The model under review builds one solid part; all positions refer to its coordinate system, in mm. A direction names the side the tool comes from. Round coordinates to 2 decimals unless told otherwise and drop trailing zeros. Order: outer loops, then holes, each group sorted by start corner. A loop starts at its lowest first (then second) coordinate and runs counter-clockwise, first axis right, second up. Notation, with made-up numbers: M 17,26.5 L 62,26.5 A20 cw 62,55.5 Z; hole C -32.75,77 d7. An arc over 180 degrees is marked long. Use a Markdown table: item, result. Add a question column.
1. Insertion check: P1, Ø1, axis at x = -1, z = 0.5, coming from the +Y side; P2, Ø1, axis at x = 33.5, z = -0.5, coming from the +Y side. Each pin has a flat end and moves straight along its axis. Give the tip position at first contact, or say it passes through.
2. Consider section B-B on x = 10.5. State the section outline as (y, z) points.
3. For faces 4 (the flat face through (25, -45, 0)), 5 (the flat face through (45, -50, 0)), 6 (the flat face through (0, 42, 0)), list the 3-axis set-ups (+Z, -Z, +X, -X, +Y, -Y) from which the entire face can be reached by the end or side of a thin tool; tool diameter is ignored.
4. Consider section A-A on z = -0.7. State the section outline as (x, y) points, then the cut area to 3 significant figures.
5. To check wall thickness, follow probe 1 along X at (y, z) = (30.5, -1); probe 2 along Y at (x, z) = (9, -0.9); probe 3 along Y at (x, z) = (2, -0.3). State the ranges of each line that lie inside material, in increasing order.
6. Consider section C-C on y = 19. State the section outline as (x, z) points, then the cut area to 4 significant figures.
7. The part is to be moulded in two halves that separate along Y. For faces 1 (the flat face through (4, 45, 0)), 2 (the flat face through (5, -1, 0)), 3 (the flat face through (3.146, 43.479, -0.022)), say which applies: +Y half, -Y half, draft (parallel to the pull), parting line (faces both ways), or undercut.
Autodesk Inventor part; units mm, degrees
ref_plane "YZ Plane" through (0, 0, 0) normal (1, 0, 0) x (0, 1, 0)
ref_plane "XZ Plane" through (0, 0, 0) normal (0, 1, 0) x (-1, 0, 0)
ref_plane "XY Plane" through (0, 0, 0) normal (0, 0, 1) x (1, 0, 0)
sketch "Sketch1" plane through (0, 0, 0) normal (0, 0, 1) x (1, 0, 0)
  line L0 (5, -45) -> (5, 45)
  line L1 (-5, 45) -> (-5, -55)
  line L2 (-5, -55) -> (45, -55)
  line L3 (45, -55) -> (45, -45)
  line L4 (45, -45) -> (5, -45)
  line L5 (0, 45) -> (0, 42) construction
  line L6 (0, 42) -> (4, 42)
  line L7 (4, 42) -> (0, 42)
  line L8 (4, 42) -> (11.2559, 42) construction
  line L9 (4, 42) -> (2.2679, 45)
  line L10 (4, 42) -> (7.4641, 42) construction
  line L11 (0, 42) -> (-4, 42)
  line L12 (-4, 42) -> (-2.2679, 45)
  line L13 (-5, 45) -> (-2.2679, 45)
  line L14 (2.2679, 45) -> (5, 45)
  line L15 (2.2679, 45) -> (-2.2679, 45) construction
  point P0 (0, 0)
  dimension "d0" = 10
  dimension "d1" = 45
  dimension "d2" = 100
  dimension "d3" = 45
  dimension "d4" = 5
  dimension "d5" = 50
  dimension "d8" = 3
  dimension "d9" = 4
  dimension "d12" = 120
  dimension "d13" = 4
  dimension "d14" = 60
  dimension "d15" = 45
  dimension "d16" = 87
  dimension "d17" = 33.7441
extrude "Extrusion1" add sketch "Sketch1" along normal mid plane 3.175
properties part number "Liu_Inital_L"
Answer block:
| question | item | result |
|---|---|---|
| 1 | P1 | y = 42 |
| 1 | P2 | y = -45 |
| 2 | outline | M -55,-1.59 L -45,-1.59 L -45,1.59 L -55,1.59 Z |
| 3 | face 4 | +Z, -Z, +X, +Y |
| 3 | face 5 | +Z, -Z, +X, +Y, -Y |
| 3 | face 6 | +Z, -Z |
| 4 | outline | M -5,-55 L 45,-55 L 45,-45 L 5,-45 L 5,45 L 2.27,45 L 4,42 L -4,42 L -2.27,45 L -5,45 Z |
| 4 | area | 1,380 mm^2 |
| 5 | probe 1 | -5 to 5 |
| 5 | probe 2 | -55 to -45 |
| 5 | probe 3 | -55 to 42 |
| 6 | outline | M -5,-1.59 L 5,-1.59 L 5,1.59 L -5,1.59 Z |
| 6 | area | 31.75 mm^2 |
| 7 | face 1 | +Y half |
| 7 | face 2 | draft |
| 7 | face 3 | undercut |
